The listing builds one solid part. Answer for the finished solid, in the listing's coordinates (mm). A direction names the side the tool comes from. Coordinates: 2 decimals unless noted, no trailing zeros. Loops run counter-clockwise (first coordinate to the right, second up) from the corner with the lowest first, then second, coordinate; pieces in that order, holes last. Notation, with made-up numbers: (3.5, 3) - (12.5, 3) arc R10 ccw to (12.5, 9) - close; hole circle Ø9 at (-18.75, -27). An arc over 180 degrees is marked (long way). Put each result on its own line as item: value.
```python
from build123d import *

# Parameters (mm, degrees)
F0_R          = 7.9375
F1_DEPTH      = 9.525
F1_DEPTH_BACK = 50.8
F2_R          = 31.75
F3_DEPTH      = 41.275
F4_R          = 15.08125
F5_DEPTH      = 101.601
F7_DEPTH      = 76.201


with BuildPart() as f1:
    # F0 (on Top) → F1 (new body, two sides)
    with BuildSketch(Plane.XY) as f1_sk:
        with BuildLine():
            Line((-323.28922, -38.1), (0, -38.1))
            ThreePointArc((0, -38.1), (38.1, 0), (0, 38.1))
            Line((0, 38.1), (-476.25, 38.1))
            Line((-476.25, 38.1), (-476.25, 0))
            ThreePointArc((-476.25, 0), (-459.600382, -18.898166), (-438.754917, -4.7625))
            ThreePointArc((-438.754917, -4.7625), (-436.495121, -1.329884), (-432.606556, 0))
            Line((-432.606556, 0), (-389.728606, 0))
            Line((-389.728606, 0), (-323.331395, -38.075815))
            Line((-323.331395, -38.075815), (-323.28922, -38.1))
        make_face()
        with Locations((-457.2, 0)):
            Circle(F0_R, mode=Mode.SUBTRACT)
        Polygon((-323.331266, -38.1), (-323.28922, -38.1), (-323.331395, -38.075815), align=None)
    extrude(amount=F1_DEPTH)
    extrude(f1_sk.sketch, amount=-F1_DEPTH_BACK)

    # F2 (on face) → F3 (join)
    with BuildSketch(Plane.XY.offset(9.525)):
        Circle(F2_R)
    extrude(amount=F3_DEPTH)

    # F4 (on face) → F5 (cut, through all)
    with BuildSketch(Plane.XY.offset(50.8)):
        Circle(F4_R)
    extrude(amount=-F5_DEPTH, mode=Mode.SUBTRACT)

    # F6 (on face) → F7 (cut, through all)
    with BuildSketch(Plane(origin=(0, 38.1, 0), x_dir=(-1, 0, 0), z_dir=(0, 1, 0))):
        Polygon((-101.6, -50.8), (254, -50.8), (166.011819, 0), (-101.6, 0), align=None)
        Polygon((524.164035, 9.525), (168.564035, 9.525), (256.552216, -41.275), (524.164035, -41.275), align=None)
    extrude(amount=-F7_DEPTH, mode=Mode.SUBTRACT)


solid = f1.part
```
1) For faces 1 (the face through (-340, 9, -41.275)), 2 (the face through (-65, 1, 0)), 3 (the face through (-411, 0, -46)), determine the directions among +Z, -Z, +X, -X, +Y, -Y from which every point of the face is accessible in a straight line to the end or side of a thin tool.
Found:
face 1: +Z, -X, +Y, -Y
face 2: -Z, +X, +Y, -Y
face 3: +Z, -Z, -Y
2) Straight lines are drawn through the part: L1, parallel to Y at x = 0, z = 26; L2, parallel to Y at x = -457, z = -46; L3, parallel to Z at x = -40, y = -5.5 (3 decimals). For each, find the intervals that lie inside material, in ascending order. Write a range as [from, to].
Found:
L1: y = [-31.75, -15.08], [15.08, 31.75]
L2: y = [-19.05, -7.93], [7.93, 38.1]
L3: z = [0, 9.525]
3) The part is cut by section C-C (y = -24.5). Give the vertices of the cut face in (x, z) (3 decimals), and give its area (3 significant figures).
Found:
outline: (-347.005, -50.8) - (-254, -50.8) - (-166.012, 0) - (29.178, 0) - (29.178, 9.525) - (20.194, 9.525) - (20.194, 50.8) - (-20.194, 50.8) - (-20.194, 9.525) - (-168.564, 9.525) - (-256.552, -41.275) - (-347.005, -41.275) - close
area: 5,380 mm^2
4) The part is cut by section B-B (x = -291.5). Give the vertices of the cut face in (y, z) (3 decimals), and give its area (3 significant figures).
Found:
outline: (-38.1, -50.8) - (38.1, -50.8) - (38.1, -41.275) - (-38.1, -41.275) - close
area: 726 mm^2
5) Each of these flat-tipped pins is pushed along its axis until it touches: pin 1 (1 mm diameter, centred on x = -347, y = -27, fed in from -Z); pin 2 (8 mm diameter, centred on x = -50.5, y = 21, fed in from +Z) (3 decimals); pin 3 (6 mm diameter, centred on x = -319, y = 23, fed in from +Z) (3 decimals); pin 4 (5 mm diameter, centred on y = 12, z = 15, fed in from -X). Where does it stop, or does it pass through?
Found:
pin 1: passes through
pin 2: stops at z = 9.525
pin 3: stops at z = -41.275
pin 4: stops at x = -30.3
6) For a pull along X with two mould halves and no side action, classify faces 4 (the face through (-237, 38.1, -32)), 5 (the face through (-6.883, -30.995, 29.874)), 6 (the face through (-459.982, -18.846, -45.971)) as pulls with the +X half, pulls with the -X half, needs draft (parallel to the pull), parting line crosses it, or undercut.
Found:
face 4: needs draft
face 5: parting line crosses it
face 6: undercut
7) The part is cut by section D-D (z = -26). Give the vertices of the cut face in (x, y), and give its area (3 significant figures).
Found:
outline: (-230.1, -38.1) - (-211.05, -38.1) - (-211.05, 38.1) - (-230.1, 38.1) - close
area: 1,450 mm^2
